```python
from build123d import *

# Parameters (mm, degrees)
SKETCH1_W           = 3
SKETCH1_H           = 30
SKETCH1_W_2         = 13.5
SKETCH1_H_2         = 3
SKETCH2_R           = 17.5
BOSS_EXTRUDE1_DEPTH = 3


with BuildPart() as part:
    # Sketch1 → Revolve1 (revolve)
    with BuildSketch(Plane(origin=(0, 0, 0), x_dir=(1, 0, 0), z_dir=(0, 1, 0)), mode=Mode.PRIVATE) as revolve1_sk:
        with Locations((15, 0)):
            Rectangle(SKETCH1_W, SKETCH1_H)
        with Locations((6.75, -13.5)):
            Rectangle(SKETCH1_W_2, SKETCH1_H_2)
    revolve(revolve1_sk.sketch.rotate(Axis((0, 0, 0), (0, 0, 1)), 180), axis=Axis((0, 0, 0), (0, 0, 1)))

    # Sketch2 → Boss-Extrude1 (add)
    with BuildSketch(Plane.XY.offset(15)):
        Circle(SKETCH2_R)
    extrude(amount=BOSS_EXTRUDE1_DEPTH)


solid = part.part
```
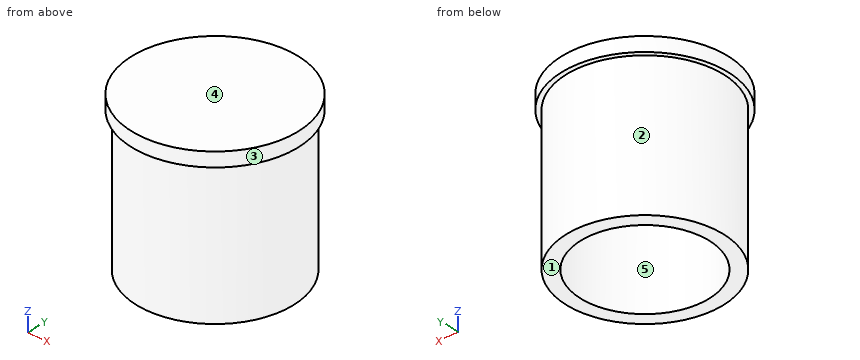
Work out the finished part from the listing and answer in its coordinate system (mm). Face numbers are marked on the shaded views. A direction names the side the tool comes from. Give positions to 0.01 mm unless a question says otherwise; leave off trailing zeros. Write each loop counter-clockwise with the first axis right and the second up, starting at its lowest first coordinate (ties: lowest second). Pieces come first, ordered by that corner, then holes. Notation, with made-up numbers: (74.25, -25.75) -> (118.25, -25.75) arc R37 cw to (118.25, 10.25) -> close; hole circle Ø2 at (9.5, -25). An arc over 180 degrees is marked (long way). Write each question's results on one line, items separated by ' | '.
1. Find section C-C on y = -0.5. Determine the outline of the cut face in (x, z).
Data:
outline: (-17.49, 15) -> (-16.49, 15) -> (-16.49, -15) -> (-13.49, -15) -> (-13.49, 12) -> (13.49, 12) -> (13.49, -15) -> (16.49, -15) -> (16.49, 15) -> (17.49, 15) -> (17.49, 18) -> (-17.49, 18) -> close
2. Straight lines are drawn through the part: L1, parallel to Y at x = 0, z = 4; L2, parallel to Z at x = 3, y = 12.5; L3, parallel to Y at x = -3, z = -3.5. For each, find the intervals that lie inside material, in ascending order.
Data:
L1: -16.5 to -13.5, 13.5 to 16.5 | L2: 12 to 18 | L3: -16.22 to -13.16, 13.16 to 16.22
3. Find section B-B on z = -9. Determine the outline of the cut face in (x, y).
Data:
outline: circle Ø33 at (0, 0); hole circle Ø27 at (0, 0)
4. A tool of negligible diameter and unlimited length cuts with its end or side. For the marked faces 1 and 2, from which of +Z, -Z, +X, -X, +Y, -Y can it reach the whole face along a straight path? Write none if from no direction.
Data:
face 1: -Z, +X, -X, +Y, -Y | face 2: -Z
5. Determine the mould class of the marked faces 3, 4 and 5 for opening direction Y: +Y half, -Y half, draft (parallel to the pull), parting line (faces both ways), or undercut.
Data:
face 3: parting line | face 4: draft | face 5: undercut
6. Each of these flat-tipped pins is pushed along its axis until it touches: pin 1 Ø4 at (x, z) = (13, -10) entering from -Y; pin 2 Ø1.5 at (x, z) = (10.5, -8.5) entering from +Y; pin 3 Ø3 at (x, z) = (0.5, 12) entering from -Y. Where does it stop, or does it pass through?
Data:
pin 1: y = -12.3 | pin 2: y = 13.31 | pin 3: y = -16.5
7. Find section A-A on x = 0. Determine the outline of the cut face in (y, z), and give its area (3 significant figures).
Data:
outline: (-17.5, 15) -> (-16.5, 15) -> (-16.5, -15) -> (-13.5, -15) -> (-13.5, 12) -> (13.5, 12) -> (13.5, -15) -> (16.5, -15) -> (16.5, 15) -> (17.5, 15) -> (17.5, 18) -> (-17.5, 18) -> close | area: 366 mm^2
8. Find section D-D on x = 15. Determine the outline of the cut face in (y, z), and give its area (3 significant figures).
Data:
outline: (-9.01, 15) -> (-6.87, 15) -> (-6.87, -15) -> (6.87, -15) -> (6.87, 15) -> (9.01, 15) -> (9.01, 18) -> (-9.01, 18) -> close | area: 467 mm^2
